The listing builds one solid part. Answer for the finished solid, in the listing's coordinates (mm). Coordinates: 2 decimals unless noted, no trailing zeros. Order: outer loops, then holes, each group sorted by start corner. A loop starts at its lowest first (then second) coordinate and runs counter-clockwise, first axis right, second up. Notation, with made-up numbers: (-4.5, 69) -> (19.5, 69) arc R26 cw to (19.5, 106) -> close; hole circle Ø11 at (-36, 16). An arc over 180 degrees is marked (long way). Return JSON: item names as keys, results as strings.
from build123d import *

# Parameters (mm, degrees)
F1_DEPTH = 15
F0_R     = 10
F2_DEPTH = 20
F3_R     = 30
F3_R_2   = 25
F4_DEPTH = 30.243643
F5_DEPTH = 51.82786
F7_W     = 79.926214
F7_H     = 10
F7_W_2   = 80.073786
F8_DEPTH = 61.82786
F9_DEPTH = 5


with BuildPart() as f1:
    # F0 (on Front) → F1 (new body, symmetric)
    with BuildSketch(Plane.XZ):
        with BuildLine():
            ThreePointArc((-95, 0), (-96.92529, -7.352004), (-102.206927, -12.816709))
            Line((-102.206927, -12.816709), (-29.805417, 6.583218))
            Line((-29.805417, 6.583218), (-29.805417, 36.82686))
            Line((-29.805417, 36.82686), (-111.573049, 14.917289))
            ThreePointArc((-111.573049, 14.917289), (-99.964955, 11.148895), (-95, 0))
        make_face()
        Polygon((-29.805417, 36.82686), (-29.805417, 6.583218), (0, 6.583218), (29.805417, 6.583218), (29.805417, 36.82686), (0, 36.82686), align=None)
        with BuildLine():
            Line((29.805417, 36.82686), (29.805417, 6.583218))
            Line((29.805417, 6.583218), (102.206927, -12.816709))
            ThreePointArc((102.206927, -12.816709), (95.788532, 4.799393), (111.573049, 14.917289))
            Line((111.573049, 14.917289), (29.805417, 36.82686))
        make_face()
    extrude(amount=F1_DEPTH, both=True)

    # F0 (on Front) → F2 (join, symmetric)
    with BuildSketch(Plane.XZ):
        with BuildLine():
            Line((-111.573049, 14.917289), (-116.096344, 13.705276))
            ThreePointArc((-116.096344, 13.705276), (-123.288101, -6.958905), (-102.206927, -12.816709))
            ThreePointArc((-102.206927, -12.816709), (-96.92529, -7.352004), (-95, 0))
            ThreePointArc((-95, 0), (-99.964955, 11.148895), (-111.573049, 14.917289))
        make_face()
        with Locations((-110, 0)):
            Circle(F0_R, mode=Mode.SUBTRACT)
        with BuildLine():
            ThreePointArc((111.573049, 14.917289), (95.788532, 4.799393), (102.206927, -12.816709))
            ThreePointArc((102.206927, -12.816709), (117.352004, -13.07471), (125, 0))
            ThreePointArc((125, 0), (122.578656, 8.171745), (116.096344, 13.705276))
            Line((116.096344, 13.705276), (111.573049, 14.917289))
        make_face()
        with Locations((110, 0)):
            Circle(F0_R, mode=Mode.SUBTRACT)
    extrude(amount=F2_DEPTH, both=True)

    # F3 (on face) → F4 (join, through all)
    with BuildSketch(Plane.XY.offset(36.82686)):
        Circle(F3_R)
        Circle(F3_R_2, mode=Mode.SUBTRACT)
    extrude(amount=-F4_DEPTH)

    # F3 (on face) → F5 (cut, through all)
    with BuildSketch(Plane.XY.offset(36.82686)):
        with BuildLine():
            ThreePointArc((25, 0), (23.717082, 7.905694), (20, 15))
            Line((20, 15), (-20, 15))
            ThreePointArc((-20, 15), (-25, 0), (-20, -15))
            Line((-20, -15), (20, -15))
            ThreePointArc((20, -15), (23.717082, -7.905694), (25, 0))
        make_face()
    extrude(amount=-F5_DEPTH, mode=Mode.SUBTRACT)

    # F7 (on offset) → F8 (cut, through all)
    with BuildSketch(Plane.XY.offset(-25)):
        with Locations((-69.963107, 0)):
            Rectangle(F7_W, F7_H)
        with Locations((70.036893, 0)):
            Rectangle(F7_W_2, F7_H)
    extrude(amount=F8_DEPTH, mode=Mode.SUBTRACT)

    # F0 (on Front) → F9 (join, symmetric)
    with BuildSketch(Plane.XZ):
        with BuildLine():
            Line((-111.573049, 14.917289), (-116.096344, 13.705276))
            ThreePointArc((-116.096344, 13.705276), (-123.288101, -6.958905), (-102.206927, -12.816709))
            ThreePointArc((-102.206927, -12.816709), (-96.92529, -7.352004), (-95, 0))
            ThreePointArc((-95, 0), (-99.964955, 11.148895), (-111.573049, 14.917289))
        make_face()
        with Locations((-110, 0)):
            Circle(F0_R, mode=Mode.SUBTRACT)
        with BuildLine():
            ThreePointArc((111.573049, 14.917289), (95.788532, 4.799393), (102.206927, -12.816709))
            ThreePointArc((102.206927, -12.816709), (117.352004, -13.07471), (125, 0))
            ThreePointArc((125, 0), (122.578656, 8.171745), (116.096344, 13.705276))
            Line((116.096344, 13.705276), (111.573049, 14.917289))
        make_face()
        with Locations((110, 0)):
            Circle(F0_R, mode=Mode.SUBTRACT)
    extrude(amount=F9_DEPTH, both=True)


solid = f1.part
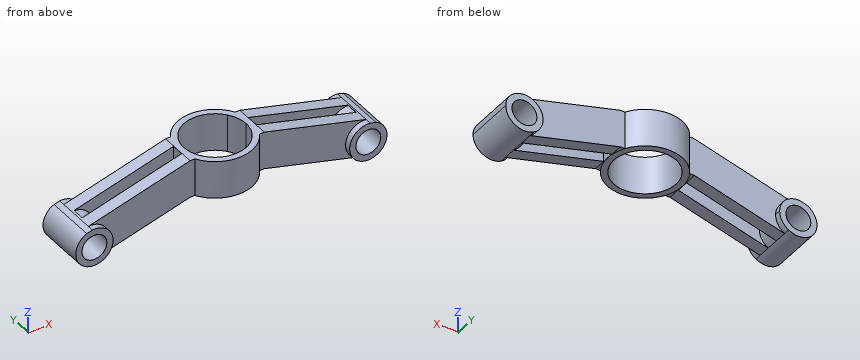
1. The part is cut by section D-D on x = -87.5. Give the vertices of the cut face in (y, z).
Answer block:
{"outline": "(-15, -8.88) -> (-5, -8.88) -> (-5, 21.37) -> (-15, 21.37) -> close; (5, -8.88) -> (15, -8.88) -> (15, 21.37) -> (5, 21.37) -> close"}
2. Consider line 1 (X direction, y = -4, z = 1); line 2 (Y direction, x = 98, z = 13.5); line 3 (Z direction, x = 110, y = -8). Determine where each line is inside the solid, lowest interval first. Write a range as from..to.
Answer block:
{"line 1": "x = -124.97..-119.95, -100.05..-95.03, 95.03..100.05, 119.95..124.97", "line 2": "y = -15..-5, 5..15", "line 3": "z = -15..-10, 10..15.34"}
3. The part is cut by section C-C on z = 31.5. Give the vertices of the cut face in (x, y), and give its area (3 significant figures).
Answer block:
{"outline": "(-49.69, -15) -> (-25.98, -15) arc R30 ccw to (25.98, -15) -> (49.69, -15) -> (49.69, -5) -> (30, -5) -> (30, 5) -> (49.69, 5) -> (49.69, 15) -> (25.98, 15) arc R30 ccw to (-25.98, 15) -> (-49.69, 15) -> (-49.69, 5) -> (-30, 5) -> (-30, -5) -> (-49.69, -5) -> close; hole (20, -15) arc R25 ccw to (25, 0) arc R25 ccw to (20, 15) arc R25 ccw (long way) to start", "area": "1,730 mm2"}
4. Each of these flat-tipped pins is pushed along its axis until it touches: pin 1 Ø24 at (x, z) = (112.5, 3) entering from +Y; pin 2 Ø15 at (x, z) = (114, -5.5) entering from -Y; pin 3 Ø2 at (y, z) = (-1.5, 17.5) entering from +X. Where does it stop, or does it pass through?
Answer block:
{"pin 1": "stops at y = 20", "pin 2": "stops at y = -20", "pin 3": "stops at x = 30"}
5. The part is cut by section A-A on x = 0. Give the vertices of the cut face in (y, z).
Answer block:
{"outline": "(-30, 6.58) -> (-25, 6.58) -> (-25, 36.83) -> (-30, 36.83) -> close; (25, 6.58) -> (30, 6.58) -> (30, 36.83) -> (25, 36.83) -> close"}
6. The part is cut by section B-B on z = -3.5. Give the number of separate pieces and of enclosed holes in the cut face, and give its area (3 significant figures).
Answer block:
{"separate pieces": "4", "enclosed holes": "0", "area": "1,950 mm2"}
